Design review of the part built by this model. Coordinates are the model's own, in mm. Face numbers are marked on the shaded views. A direction names the side the tool comes from. Round coordinates to 2 decimals unless told otherwise and drop trailing zeros. Order: outer loops, then holes, each group sorted by start corner. A loop starts at its lowest first (then second) coordinate and runs counter-clockwise, first axis right, second up.
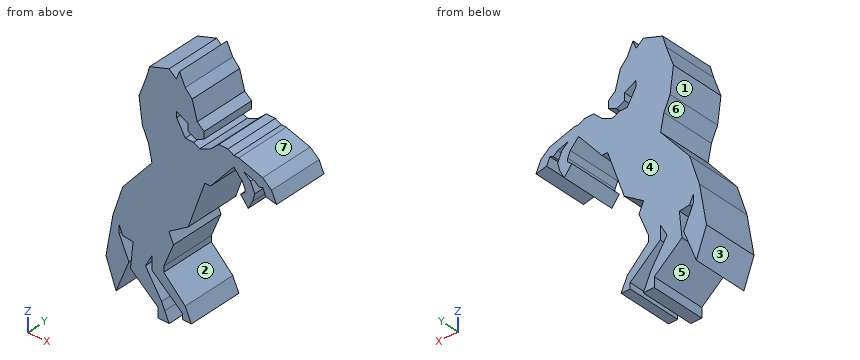
from build123d import *

# Parameters (mm, degrees)
F1_DEPTH = 25.4


# Not quite as in the source:
# - ends of sketch curves that miss each other by under 0.0002 mm in the source are joined


with BuildPart() as f1:
    # F0 (on Front) → F1 (new body)
    with BuildSketch(Plane.XZ):
        Polygon((0, 51.2815788388), (-2.6849012356, 56.9198653102), (-4.1696302487, 53.0196329049), (-7.5777377933, 55.8597221971), (-16.6846867651, 52.6580624282), (-18.2750094682, 47.2689494491), (-21.6973181814, 37.9454642534), (-20.1343216481, 26.0272607351), (-17.2047130764, 19.5402652025), (-15.6613234345, 11.8683064511), (-29.3124747088, -4.5130769722), (-33.9270979166, -18.5791757945), (-37.2212677423, -37.4857979189), (-32.480597056, -50.5585558089), (-26.4811083451, -35.4206826298), (-31.0107059295, -25.3908514852), (-31.0107059295, -21.6304793835), (-29.3124747088, -25.3908514852), (-24.4753230363, -25.888632983), (-25.7045285945, -37.8333391404), (-12.6969534904, -48.6729838072), (-12.6969534904, -53.2361328939), (-7.5467102784, -53.2361328939), (-9.6074856576, -48.6729838072), (-11.097422801, -45.3738346696), (-18.6685893591, -33.5405004938), (-15.5289131012, -27.6335775852), (-15.5289131012, -34.1437415194), (-1.3548218412, -45.9554828703), (-1.3548218412, -48.6729838072), (2.8690039134, -48.6729838072), (0, -42.3201844096), (-10.079539381, -32.4321724474), (-10.079539381, -29.8147555441), (-5.5140842237, -18.5791757945), (-7.6782507822, -13.7870889157), (1.4005823759, -7.7723623253), (9.2310756445, 14.5376751978), (11.9198445967, 14.5376751978), (22.8343526097, 27.6350863278), (26.7602472754, 23.3975637498), (28.004777182, 20.64181678), (28.004777182, 19.005872948), (26.0269176215, 17.4214001745), (29.5830273071, 12.9823932965), (31.7011885345, 16.9674586505), (32.6957959123, 20.64181678), (30.6835759384, 25.0974502414), (27.5022275746, 27.7485735714), (32.7634411399, 26.0272607351), (34.7447489485, 24.3761710855), (36.341868341, 25.0974502414), (37.8633029759, 21.7285566032), (42.8623110056, 20.64181678), (40.5427415461, 25.7263357936), (36.341868341, 29.2270630598), (25.148447603, 32.5854149557), (22.8343526097, 32.5854149557), (20.0345981866, 34.0735539794), (15.7886892557, 34.0735539794), (11.8005704135, 30.2826426923), (6.8094845357, 28.1176646778), (3.9549916983, 29.6348985285), (0, 29.6348985285), (-4.0098810568, 36.5146324039), (-4.0098810568, 39.3167249858), (1.2619188055, 36.5146324039), (1.2619188055, 33.1852734089), (5.1013175398, 31.4132459462), (8.8601689786, 33.1852734089), (8.8601689786, 36.5146324039), (5.6382901967, 39.1995310783), (3.2218813431, 47.7912090719), align=None)
    extrude(amount=F1_DEPTH)


solid = f1.part
1) To check wall thickness, follow line 1 along X through (y, z) = (-14.5, 24.5); line 2 along Z through (x, y) = (0, -2.25); line 3 along X through (y, z) = (-1.25, 17.5). State the ranges of each line that lie inside material, in increasing order.
Results:
line 1: x = -19.44 to 20.22, 25.74 to 30.95, 34.6 to 35.02, 36.61 to 41.1
line 2: z = -48.67 to -42.32, -8.7 to 29.63, 37.19 to 51.28
line 3: x = -16.79 to 14.39, 26.13 to 31.85
2) Take a section at A-A on z = 42. Give the boundary of the cut face in (x, y), plus the area to 3 significant figures.
Results:
outline: (-20.21, -25.4) - (4.85, -25.4) - (4.85, 0) - (-20.21, 0) - close
area: 637 mm2
3) For the marked faces 1, 2 and 3, list the 3-axis set-ups (+Z, -Z, +X, -X, +Y, -Y) from which the entire face can be reached by the end or side of a thin tool; tool diameter is ignored.
Results:
face 1: -X, +Y, -Y
face 2: +X, +Y, -Y
face 3: -Z, -X, +Y, -Y
4) Take a section at B-B on z = 3.5. Give the boundary of the cut face in (x, y), plus the area to 3 significant figures.
Results:
outline: (-22.63, -25.4) - (5.36, -25.4) - (5.36, 0) - (-22.63, 0) - close
area: 711 mm2
5) Clearance check with flat-ended pins moving along their axes: P1, Ø6, axis at x = 20.5, y = -16.5, coming from the -Z side; P2, Ø3, axis at y = -13, z = 38.5, coming from the -X side; P3, Ø1.3, axis at x = 1, y = -18, coming from the -Z side. State where each tip first meets the part, or that it passes through.
Results:
P1: stops at z = 21.23
P2: stops at x = -21.7
P3: stops at z = -48.67
6) The part is to be moulded in two halves that separate along X. For the marked faces 4, 5, 6 and 7, say which applies: released by +X, released by -X, zero draft, split by the parting line, or undercut.
Results:
face 4: zero draft
face 5: undercut
face 6: released by -X
face 7: released by +X
